Source: CAD feature listing. Evaluate the final solid. Frame: model axes, mm. A direction names the side the tool comes from. Coordinates: 2 decimals unless noted, no trailing zeros. Order: outer loops, then holes, each group sorted by start corner. A loop starts at its lowest first (then second) coordinate and runs counter-clockwise, first axis right, second up.
```python
from build123d import *

# Parameters (mm, degrees)
SKETCH2_W                = 10
SKETCH2_H                = 100
BOSS_EXTRUDE1_DEPTH      = 10
FILLET1_R                = 5
CUT_EXTRUDE1_DEPTH       = 3
CUT_EXTRUDE2_START       = 7
SKETCH3_2_W              = 10
SKETCH3_2_H              = 9
CUT_EXTRUDE2_DEPTH       = 3
CUT_EXTRUDE4_START       = -4
CUT_EXTRUDE4_DEPTH       = 56.23475383
SKETCH7_R                = 1.5
CUT_EXTRUDE5_DEPTH       = 51.734603576
BOSS_EXTRUDE2_DEPTH      = 7
BOSS_EXTRUDE2_DEPTH_BACK = 7
SKETCH9_W                = 15
SKETCH9_H                = 70
FILLET3_R                = 7


with BuildPart() as part:
    # Sketch2 → Boss-Extrude1 (new body)
    with BuildSketch(Plane.XY):
        Rectangle(SKETCH2_W, SKETCH2_H)
    extrude(amount=BOSS_EXTRUDE1_DEPTH)

    # Fillet1
    fillet1_edges = [part.edges().sort_by_distance(p)[0] for p in [
        (-5, 0, 0),
        (5, 0, 0),
        (5, 0, 10),
        (-5, 0, 10),
    ]]
    fillet(fillet1_edges, radius=FILLET1_R - 0.0001)  # a hair under: the kernel refuses the full size

    # Sketch3 → Cut-Extrude1 (cut)
    with BuildSketch(Plane.XY):
        with BuildLine():
            Line((-5, -41), (-4.5, -45.5))
            ThreePointArc((-4.5, -45.5), (0, -50), (4.5, -45.5))
            Line((4.5, -45.5), (5, -41))
            Line((5, -41), (-5, -41))
        make_face()
        with BuildLine():
            Line((0, -50), (5, -50))
            Line((5, -50), (5, -41))
            Line((5, -41), (4.5, -45.5))
            ThreePointArc((4.5, -45.5), (3.181980515, -48.681980515), (0, -50))
        make_face()
        with BuildLine():
            Line((-5, -50), (0, -50))
            ThreePointArc((0, -50), (-3.181980515, -48.681980515), (-4.5, -45.5))
            Line((-4.5, -45.5), (-5, -41))
            Line((-5, -41), (-5, -50))
        make_face()
    cut_extrude1 = extrude(amount=CUT_EXTRUDE1_DEPTH, mode=Mode.SUBTRACT)

    # Sketch3<2> → Cut-Extrude2 (cut)
    with BuildSketch(Plane.XY.offset(CUT_EXTRUDE2_START)):
        with Locations((0, -45.5)):
            Rectangle(SKETCH3_2_W, SKETCH3_2_H)
    cut_extrude2 = extrude(amount=CUT_EXTRUDE2_DEPTH, mode=Mode.SUBTRACT)

    # Mirror1: Cut-Extrude1, Cut-Extrude2 across plane
    add(cut_extrude1.mirror(Plane.ZX), mode=Mode.SUBTRACT)
    add(cut_extrude2.mirror(Plane.ZX), mode=Mode.SUBTRACT)

    # Sketch3<4> → Cut-Extrude4 (cut)
    with BuildSketch(Plane.XY.offset(CUT_EXTRUDE4_START)):
        with BuildLine():
            Line((0, -50), (5, -50))
            Line((5, -50), (5, -41))
            Line((5, -41), (4.5, -45.5))
            ThreePointArc((4.5, -45.5), (3.181980515, -48.681980515), (0, -50))
        make_face()
        with BuildLine():
            Line((-5, -50), (0, -50))
            ThreePointArc((0, -50), (-3.181980515, -48.681980515), (-4.5, -45.5))
            Line((-4.5, -45.5), (-5, -41))
            Line((-5, -41), (-5, -50))
        make_face()
    cut_extrude4 = extrude(amount=CUT_EXTRUDE4_DEPTH, mode=Mode.SUBTRACT)

    # Sketch7 → Cut-Extrude5 (cut, through all)
    with BuildSketch(Plane(origin=(0, 0, 3), x_dir=(-1, 0, 0), z_dir=(0, 0, -1))):
        with Locations((0, -45.5)):
            Circle(SKETCH7_R)
    cut_extrude5 = extrude(amount=-CUT_EXTRUDE5_DEPTH, mode=Mode.SUBTRACT)

    # Mirror3: Cut-Extrude5 across plane
    add(cut_extrude5.mirror(Plane.ZX), mode=Mode.SUBTRACT)

    # Mirror4: Cut-Extrude4 across plane
    add(cut_extrude4.mirror(Plane.ZX), mode=Mode.SUBTRACT)

    # Sketch9 → Boss-Extrude2 (add, two sides: drawn at the far end of the back side and taken through both)
    with BuildSketch(Plane.XY.offset(5).offset(-BOSS_EXTRUDE2_DEPTH_BACK)):
        Rectangle(SKETCH9_W, SKETCH9_H)
    extrude(amount=BOSS_EXTRUDE2_DEPTH + BOSS_EXTRUDE2_DEPTH_BACK)

    # Fillet3
    fillet3_edges = [part.edges().sort_by_distance(p)[0] for p in [
        (-7.5, 0, 12),
        (7.5, 0, 12),
        (7.5, 0, -2),
        (-7.5, 0, -2),
    ]]
    fillet(fillet3_edges, radius=FILLET3_R - 0.0001)  # a hair under: the kernel refuses the full size


solid = part.part
```
Q1. Pin query (flat end, axial travel): P1, Ø4, axis at x = -4, y = -28.5, coming from the +Z side; P2, Ø2, axis at y = -4.5, z = 0, coming from the +X side; P3, Ø4, axis at y = -0.5, z = 0, coming from the +X side. Return the tip coordinate at first contact, or that it passes through.
Solutions:
P1: stops at z = 11.84
P2: stops at x = 6.24
P3: stops at x = 6.82
Q2. Pull-direction query (Y, two-part tool) for faces 1 (the cylindrical face through (0, 47, 5)), 2 (the flat face through (4.7, -43.7, 5)), 3 (the flat face through (-1, -44, 3)); classes: pulls with the +Y half, pulls with the -Y half, needs draft (parallel to the pull), parting line crosses it, or undercut.
Solutions:
face 1: undercut
face 2: pulls with the -Y half
face 3: needs draft
Q3. Material intervals for line 1 along Y through (x, z) = (0, 4.1); line 2 along X through (y, z) = (45.5, 4.85); line 3 along Y through (x, z) = (2.5, -1.25), sorted ascending.
Solutions:
line 1: y = -50 to -47, -44 to 44, 47 to 50
line 2: x = -4.5 to -1.5, 1.5 to 4.5
line 3: y = -35 to 35
Q4. Section query B-B on z = 1. Output: boundary loops of the cut face in (x, y), plus the area to 3 significant figures.
Solutions:
outline: (-6.24, -35) - (-3, -35) - (-3, -41) - (3, -41) - (3, -35) - (6.24, -35) - (6.24, 35) - (3, 35) - (3, 41) - (-3, 41) - (-3, 35) - (-6.24, 35) - close
area: 946 mm2
Q5. Set-up query: faces 4 (the flat face through (-1, 44, 7)), 5 (the cylindrical face through (4, -39, 8)), 6 (the cylindrical face through (4, -39, 2)), 7 (the cylindrical face through (-4, 38, 2)), 8 (the flat face through (0, -41, 2)). Return all of +Z, -Z, +X, -X, +Y, -Y with unobstructed straight access to the full face (end or side cutting, diameter ignored); none if empty.
Solutions:
face 4: +Z, +X, -X, +Y
face 5: +Z, +X, -Y
face 6: -Z, +X, -Y
face 7: -Z, -X, +Y
face 8: -Z, +X, -X, -Y
